Model file for the job. Use its own axes, mm. A direction names the side the tool comes from. Round coordinates to 2 decimals unless told otherwise and drop trailing zeros. Order: outer loops, then holes, each group sorted by start corner. A loop starts at its lowest first (then second) coordinate and runs counter-clockwise, first axis right, second up. Notation, with made-up numbers: (53.5, 43.5) - (82.5, 43.5) arc R20 cw to (82.5, 68.5) - close; hole circle Ø8 at (-24.75, -36.75). An arc over 180 degrees is marked (long way). Answer as CSV lines item,"result". Start each with the question number.
1. 3-axis set-ups, long thin cutter, end or side, ignore diameter. For faces 1 (the face through (0, 0, 0)), 2 (the face through (0, 29, 2.165)), 3 (the face through (0.54, 9.86, 2.44)): which of +Z, -Z, +X, -X, +Y, -Y reach the whole face in a straight line?
2. Band-saw the part on A-A on x = 0. List the corners of the cut face in (y, z), then the cut area to 3 significant figures.
3. Wall check: line 1 along X through (y, z) = (23.25, 0.25); line 2 along Z through (x, y) = (-2, 28); line 3 along Y through (x, z) = (1, 2). Give the ranges that are in metal, low to high. Write a range as [from, to].
4. Pin check, flat tips, straight feed: pin 1 Ø5 at (x, y) = (0.5, 6.5) entering from -Z; pin 2 Ø2 at (x, z) = (2, -3.5) entering from -Y; pin 3 Ø6 at (y, z) = (11.5, 1) entering from -X. Stop position of each tip, or through.
5. Pull direction Z, two halves, no side cores. Call faces 4 (the face through (-1.88, 28.52, -1.07)), 5 (the face through (2, 20, 2)), 6 (the face through (-1.08, 24.19, -4.88)): released by +Z, released by -Z, zero draft, split by the parting line, or undercut.
6. Band-saw the part on B-B on y = 5.5. List the corners of the cut face in (x, z).
Autodesk Inventor part; units mm, degrees
ref_plane "YZ Plane" through (0, 0, 0) normal (1, 0, 0) x (0, 1, 0)
ref_plane "XZ Plane" through (0, 0, 0) normal (0, 1, 0) x (-1, 0, 0)
ref_plane "XY Plane" through (0, 0, 0) normal (0, 0, 1) x (1, 0, 0)
sketch "Sketch1" plane through (0, 0, 0) normal (0, 1, 0) x (-1, 0, 0)
  circle A0 centre (0, 0) radius 2.5
  dimension "d0" = 5
extrude "Extrusion1" add sketch "Sketch1" along normal blind 20
sketch "Sketch2" plane through (0, 20, 0) normal (0, 1, 0) x (1, 0, 0)
  circle A0 centre (0, 0) radius 5
extrude "Extrusion2" add sketch "Sketch2" along normal blind 10
sketch "Sketch3" plane through (0, 30, 0) normal (0, 1, 0) x (1, 0, 0)
  circle A0 centre (0, 0) radius 2.5
  line L0 (2.5, 0) -> (1.25, -2.1651)
  line L1 (1.25, -2.1651) -> (-1.25, -2.1651)
  line L2 (-1.25, -2.1651) -> (-2.5, 0)
  line L3 (-2.5, 0) -> (-1.25, 2.1651)
  line L4 (-1.25, 2.1651) -> (1.25, 2.1651)
  line L5 (1.25, 2.1651) -> (2.5, 0)
fillet "Fillet1" radius 1.5 1 edges at (-5, 30, 0)
extrude "Extrusion3" cut sketch "Sketch3" against normal blind 3 contours L0 L1 L2 L3 L4 L5
properties part number "35mm_bolt"
Reply:
1,face 1,"+Z, -Z, +X, -X, -Y"
1,face 2,"+Y"
1,face 3,"-Y"
2,outline,"(0, -2.5) - (20, -2.5) - (20, -5) - (28.5, -5) arc R1.5 ccw to (30, -3.5) - (30, -2.17) - (27, -2.17) - (27, 2.17) - (30, 2.17) - (30, 3.5) arc R1.5 ccw to (28.5, 5) - (20, 5) - (20, 2.5) - (0, 2.5) - close"
2,area,"186 mm2"
3,line 1,"x = [-4.99, 4.99]"
3,line 2,"z = [-4.58, -0.87], [0.87, 4.58]"
3,line 3,"y = [0, 27]"
4,pin 1,"stops at z = -2.5"
4,pin 2,"stops at y = 20"
4,pin 3,"stops at x = -2.5"
5,face 4,"undercut"
5,face 5,"zero draft"
5,face 6,"split by the parting line"
6,outline,"circle Ø5 at (0, 0)"
